from build123d import *

# Parameters (mm, degrees)
ESQUISSE1_R                                     = 11.25
BOSS_EXTRU_1_DEPTH                              = 2
ESQUISSE8_R                                     = 11.25
BOSS_EXTRU_2_DEPTH                              = 3
ESQUISSE15_W                                    = 21.34
ESQUISSE15_H                                    = 21.34
BOSS_EXTRU_3_DEPTH                              = 2
ESQUISSE14_R                                    = 5
ENL_V_MAT_EXTRU_3_DEPTH                         = 6
D_GAGEMENT_M21_D                                = 3.5
ENL_V_MAT_EXTRU_11_DEPTH                        = 3
CONG_1_R                                        = 5
ESQUISSE20_R                                    = 6.103277808
ESQUISSE20_R_2                                  = 5
BOSS_EXTRU_5_DEPTH                              = 3
CONG_3_R                                        = 2.5
CHAMBRAGE_POUR_VIS_T_TE_CYLINDRIQUE_D           = 2.5
CHAMBRAGE_POUR_VIS_T_TE_CYLINDRIQUE_CBORE_D     = 4.5
CHAMBRAGE_POUR_VIS_T_TE_CYLINDRIQUE_CBORE_DEPTH = 3.3


with BuildPart() as part:
    # Esquisse1 → Boss.-Extru.1 (new body)
    with BuildSketch(Plane(origin=(0, 0, 0), x_dir=(1, 0, 0), z_dir=(0, 1, 0))):
        Circle(ESQUISSE1_R)
    extrude(amount=BOSS_EXTRU_1_DEPTH)

    # Esquisse8 → Boss.-Extru.2 (add)
    with BuildSketch(Plane.XZ):
        Circle(ESQUISSE8_R)
    extrude(amount=BOSS_EXTRU_2_DEPTH)

    # Esquisse15 → Boss.-Extru.3 (add)
    with BuildSketch(Plane(origin=(0, 2, 0), x_dir=(1, 0, 0), z_dir=(0, 1, 0))):
        Rectangle(ESQUISSE15_W, ESQUISSE15_H)
    extrude(amount=-BOSS_EXTRU_3_DEPTH)

    # Esquisse14 → Enlèv. mat.-Extru.3 (cut)
    with BuildSketch(Plane.XZ.offset(3)):
        Circle(ESQUISSE14_R)
    extrude(amount=-ENL_V_MAT_EXTRU_3_DEPTH, mode=Mode.SUBTRACT)

    # Dégagement M21 (through all)
    with Locations(Plane(origin=(0, 2, 0), x_dir=(1, 0, 0), z_dir=(0, 1, 0))):
        with Locations((6.92, -6.92), (-6.92, -6.92), (-6.92, 6.92), (6.92, 6.92)):
            Hole(D_GAGEMENT_M21_D / 2)

    # Esquisse18 → Enlèv. mat.-Extru.11 (cut)
    with BuildSketch(Plane.XZ):
        Polygon((-3.5, -10.67), (-3.5, -5), (3.5, -5), (3.5, -10.67), (10.67, -10.67), (10.67, -3.5), (5, -3.5), (5, 3.5), (10.67, 3.5), (10.67, 10.67), (3.5, 10.67), (3.5, 5), (-3.5, 5), (-3.5, 10.67), (-10.67, 10.67), (-10.67, 3.5), (-5, 3.5), (-5, -3.5), (-10.67, -3.5), (-10.67, -10.67), align=None)
    extrude(amount=ENL_V_MAT_EXTRU_11_DEPTH, mode=Mode.SUBTRACT)

    # Congé1
    cong_1_edges = [part.edges().sort_by_distance(p)[0] for p in [
        (-10.67, 1, 10.67),
        (-10.67, 1, -10.67),
        (10.67, 1, -10.67),
        (10.67, 1, 10.67),
    ]]
    fillet(cong_1_edges, radius=CONG_1_R)

    # Esquisse20 → Boss.-Extru.5 (add)
    with BuildSketch(Plane.XZ):
        Circle(ESQUISSE20_R)
        Circle(ESQUISSE20_R_2, mode=Mode.SUBTRACT)
    extrude(amount=BOSS_EXTRU_5_DEPTH)

    # Congé3
    cong_3_edges = [part.edges().sort_by_distance(p)[0] for p in [
        (-5, -1.5, 3.5),
        (-3.5, -1.5, -5),
        (5, -1.5, -3.5),
        (3.5, -1.5, 5),
        (-5, -1.5, -3.5),
        (3.5, -1.5, -5),
        (5, -1.5, 3.5),
        (-3.5, -1.5, 5),
    ]]
    fillet(cong_3_edges, radius=CONG_3_R)

    # Chambrage pour vis à tête cylindrique à 6 pans creux (ou vis CHC) M21 (through all)
    with Locations(Plane(origin=(0, 2, 0), x_dir=(1, 0, 0), z_dir=(0, 1, 0))):
        with Locations((-8, 0), (0, -8), (8, 0), (0, 8)):
            CounterBoreHole(CHAMBRAGE_POUR_VIS_T_TE_CYLINDRIQUE_D / 2, CHAMBRAGE_POUR_VIS_T_TE_CYLINDRIQUE_CBORE_D / 2, CHAMBRAGE_POUR_VIS_T_TE_CYLINDRIQUE_CBORE_DEPTH)


solid = part.part
The listing builds one solid part. Answer for the finished solid, in the listing's coordinates (mm). A direction names the side the tool comes from. Coordinates: 2 decimals unless noted, no trailing zeros. Order: outer loops, then holes, each group sorted by start corner. A loop starts at its lowest first (then second) coordinate and runs counter-clockwise, first axis right, second up.
Q1. Given P1, Ø1.6, axis at y = 1.5, z = -4.5, coming from the +X side; P2, Ø1.6, axis at x = 4.5, y = 1, coming from the -Z side; P3, Ø1.5, axis at y = -2, z = 7.5, coming from the -X side, each flat-ended and moving along its own axis, determine where each tip first touches the part or whether it passes through.
Q2. Which of the six approach directions +Z, -Z, +X, -X, +Y, -Y give full straight-line access (tool end or side, diameter ignored) to faces 4 (the face through (-5, 1, 10.67)), 5 (the face through (3.702, -1.521, 5.18)), 6 (the face through (-5, 1, -10.67)), 7 (the face through (1, -1.3, -7))?
Q3. A cutting plane is placed at B-B, the plane z = 8. Write down the section's boundary in (x, y).
Q4. For a pull along Z with two mould halves and no side action, classify faces 1 (the face through (-9.17, 0.99, -9.24)), 2 (the face through (-0.29, 0.37, 5.77)), 3 (the face through (-8, -1, 3.5)) as pulls with the +Z half, pulls with the -Z half, needs draft (parallel to the pull), parting line crosses it, or undercut.
Q5. Consider line 1 (Z direction, x = 7.5, y = 1.1); line 2 (X direction, y = 0.25, z = 8); line 3 (Y direction, x = 7.25, z = -2). Determine where each line is inside the solid, lowest interval first.
Q6. A cutting plane is placed at A-A, the plane y = 0.75. State how many separate pieces and enclosed holes the cut face has, and give its area (3 significant figures).
Answers follow:
1. P1: stops at x = 10.67
1. P2: stops at z = -10.67
1. P3: stops at x = -3.5
2. face 4: +Z, -X, +Y, -Y
2. face 5: +X, -Y
2. face 6: -Z, -X, +Y, -Y
2. face 7: +Y
3. outline: (-10.09, 0) - (-8.3, 0) - (-8.3, 2) - (-10.09, 2) - close; (-5.54, 0) - (-3.5, 0) - (-3.5, -3) - (-1.25, -3) - (-1.25, -1.3) - (-2.25, -1.3) - (-2.25, 2) - (-5.54, 2) - close; (1.25, -3) - (3.5, -3) - (3.5, 0) - (5.54, 0) - (5.54, 2) - (2.25, 2) - (2.25, -1.3) - (1.25, -1.3) - close; (8.3, 0) - (10.09, 0) - (10.09, 2) - (8.3, 2) - close
4. face 1: pulls with the -Z half
4. face 2: undercut
4. face 3: pulls with the +Z half
5. line 1: z = -10.32 to -8.57, -5.27 to -2.19, 2.19 to 5.27, 8.57 to 10.32
5. line 2: x = -10.09 to -8.3, -5.54 to -2.25, 2.25 to 5.54, 8.3 to 10.09
5. line 3: y = -3 to -1.3
6. separate pieces: 1
6. enclosed holes: 9
6. area: 264 mm2
